```python
from build123d import *

# Parameters (mm, degrees)
F0_W           = 16
F0_H           = 16
F1_DEPTH       = 1
F2_W           = 8
F2_H           = 8
F2_W_2         = 5
F2_H_2         = 5
F3_DEPTH       = 2.5
F4_SIZE        = 1
F5_DEPTH       = 5
F6_DEPTH       = 5
F7_DEPTH       = 5
F8_DEPTH       = 5
F9_SIZE2       = 2
F9_SIZE        = 5
F10_W          = 3
F10_H          = 1.5
F11_DEPTH      = 8.001
F11_DEPTH_BACK = 8.001
F12_W          = 3
F12_H          = 1.5
F13_DEPTH      = 8.001
F13_DEPTH_BACK = 8.001
F14_R          = 1


with BuildPart() as f1:
    # F0 (on Top) → F1 (new body)
    with BuildSketch(Plane.XY):
        Rectangle(F0_W, F0_H)
    extrude(amount=F1_DEPTH)

    # F2 (on face) → F3 (join)
    with BuildSketch(Plane.XY.offset(1)):
        Rectangle(F2_W, F2_H)
        Rectangle(F2_W_2, F2_H_2, mode=Mode.SUBTRACT)
    extrude(amount=F3_DEPTH)

    # F4
    f4_edges = [f1.edges().sort_by_distance(p)[0] for p in [
        (4, 4, 2.25),
        (-4, 4, 2.25),
        (-4, -4, 2.25),
        (4, -4, 2.25),
    ]]
    chamfer(f4_edges, length=F4_SIZE)

    # F5 (add): a face of the model
    f5_faces = [f1.faces().sort_by_distance(p)[0] for p in [
        (-3.5, -3.5, 2.25),
    ]]
    extrude(f5_faces, amount=F5_DEPTH)

    # F6 (add): a face of the model
    f6_faces = [f1.faces().sort_by_distance(p)[0] for p in [
        (3.5, -3.5, 2.25),
    ]]
    extrude(f6_faces, amount=F6_DEPTH)

    # F7 (add): a face of the model
    f7_faces = [f1.faces().sort_by_distance(p)[0] for p in [
        (-3.5, 3.5, 2.25),
    ]]
    extrude(f7_faces, amount=F7_DEPTH)

    # F8 (add): a face of the model
    f8_faces = [f1.faces().sort_by_distance(p)[0] for p in [
        (3.5, 3.5, 2.25),
    ]]
    extrude(f8_faces, amount=F8_DEPTH)

    # F9
    f9_edges = [f1.edges().sort_by_distance(p)[0] for p in [
        (-7.035534, 7.035534, 3.5),
        (-7.035534, -7.035534, 3.5),
        (7.035534, -7.035534, 3.5),
        (7.035534, 7.035534, 3.5),
    ]]
    f9_side = f1.faces().sort_by_distance((0, 3.786863, 3.5))[0]
    chamfer(f9_edges, length=F9_SIZE, length2=F9_SIZE2, reference=f9_side)

    # F10 (on Front) → F11 (cut, two sides)
    with BuildSketch(Plane.XZ) as f11_sk:
        with Locations((0, 1.75)):
            Rectangle(F10_W, F10_H)
    extrude(amount=-F11_DEPTH, mode=Mode.SUBTRACT)
    extrude(f11_sk.sketch, amount=F11_DEPTH_BACK, mode=Mode.SUBTRACT)

    # F12 (on Right) → F13 (cut, two sides)
    with BuildSketch(Plane.YZ) as f13_sk:
        with Locations((0, 1.75)):
            Rectangle(F12_W, F12_H)
    extrude(amount=-F13_DEPTH, mode=Mode.SUBTRACT)
    extrude(f13_sk.sketch, amount=F13_DEPTH_BACK, mode=Mode.SUBTRACT)

    # F14
    f14_edges = [f1.edges().sort_by_distance(p)[0] for p in [
        (-2.5, 2.5, 2.25),
        (-2.5, -2.5, 2.25),
        (2.5, 2.5, 2.25),
        (2.5, -2.5, 2.25),
        (8, -8, 0.5),
        (8, 8, 0.5),
        (-8, -8, 0.5),
        (-8, 8, 0.5),
    ]]
    fillet(f14_edges, radius=F14_R)


solid = f1.part
```
Could you check a few things on this model? Use its own coordinates, in mm. A direction names the side the tool comes from. Give positions to 0.01 mm unless a question says otherwise; leave off trailing zeros. Loops run counter-clockwise (first coordinate to the right, second up) from the corner with the lowest first, then second, coordinate; pieces in that order, holes last. Notation, with made-up numbers: (71, 50) -> (113, 50) arc R18 ccw to (113, 82) -> close; hole circle Ø1 at (54, -40). An arc over 180 degrees is marked (long way). Put each result on its own line as item: value.
(1) Imagine slicing it at D-D on y = -3.5. Write out the boundary of the cut face in (x, z).
Computed:
outline: (-8, 0) -> (8, 0) -> (8, 1) -> (4.5, 1) -> (4.5, 3.22) -> (3.5, 3.5) -> (-3.5, 3.5) -> (-4.5, 3.22) -> (-4.5, 1) -> (-8, 1) -> close; hole (-1.5, 1) -> (1.5, 1) -> (1.5, 2.5) -> (-1.5, 2.5) -> close
(2) I'm going to push flat-ended pins straight in: pin 1 Ø0.8 at (x, z) = (1.5, 3) entering from +Y; pin 2 Ø1 at (x, y) = (5, 1) entering from +Z; pin 3 Ø0.8 at (x, z) = (3, 2) entering from +Y. Where does each tip first touch, or does it pass through?
Computed:
pin 1: y = 4
pin 2: z = 1
pin 3: y = 4.4
(3) Imagine slicing it at C-C on z = 2.2. State how many separate pieces and enclosed holes the cut face has, plus the area to 3 significant figures.
Computed:
separate pieces: 4
enclosed holes: 0
area: 38.2 mm^2
(4) Thinking about a two-plate mould opening in Y: for faces 4 (the face through (7.715, -7.699, 0.507)), 5 (the face through (0, 4, 3)), 6 (the face through (-3, 1.5, 2)), 7 (the face through (8, -0.1, 0.5)), which applies, pulls with the +Y half, pulls with the -Y half, needs draft (parallel to the pull), parting line crosses it, or undercut?
Computed:
face 4: pulls with the -Y half
face 5: pulls with the +Y half
face 6: undercut
face 7: needs draft
(5) For faces 1 (the face through (1.5, -3, 2)), 2 (the face through (7.03, 7.04, 1.25)), 3 (the face through (-2.5, 0, 3)), which set-ups out of +Z, -Z, +X, -X, +Y, -Y let a thin tool reach every point of the face, with its end or its side?
Computed:
face 1: +Y, -Y
face 2: +Z, +X, +Y
face 3: +Z
(6) Please list where these lines run through material, in increasing order: probe 1 along Z at (x, y) = (-1, 3.5); probe 2 along Z at (x, y) = (-5, 2); probe 3 along Y at (x, z) = (1.25, 3.3). Write a range as [from, to].
Computed:
probe 1: [0, 1], [2.5, 3.5]
probe 2: [0, 1]
probe 3: [-4, -2.5], [2.5, 4]
(7) Imagine slicing it at A-A on y = -1.25. Write out the boundary of the cut face in (x, z).
Computed:
outline: (-8, 0) -> (8, 0) -> (8, 1) -> (-8, 1) -> close; (-4, 2.5) -> (-2.5, 2.5) -> (-2.5, 3.5) -> (-4, 3.5) -> close; (2.5, 2.5) -> (4, 2.5) -> (4, 3.5) -> (2.5, 3.5) -> close
